Verification items for the finished model (mm, model axes). A direction names the side the tool comes from. Coordinates: 2 decimals unless noted, no trailing zeros. Order: outer loops, then holes, each group sorted by start corner. A loop starts at its lowest first (then second) coordinate and runs counter-clockwise, first axis right, second up. Notation, with made-up numbers: M 61.25,63 L 67.25,63 A21 ccw 67.25,76 Z; hole C 51.5,-37 d5. An arc over 180 degrees is marked long. Write item = value, one per line.
```python
from build123d import *

# Parameters (mm, degrees)
SKETCH1_W                  = 52
SKETCH1_H                  = 28.5
SKETCH1_R                  = 1.6
BOSS_EXTRUDE1_DEPTH        = 1.6
FILLET1_R                  = 2
SKETCH2_W                  = 6
SKETCH2_H                  = 8
BOSS_EXTRUDE2_DEPTH        = 2.6
SKETCH3_W                  = 26.5
SKETCH3_H                  = 18.5
BOSS_EXTRUDE3_DEPTH        = 0.9
SKETCH4_W                  = 19
SKETCH4_H                  = 18.5
BOSS_EXTRUDE4_DEPTH        = 2.4
SKETCH5_W                  = 4.480247742
SKETCH5_H                  = 2.767211841
SKETCH5_H_2                = 2.398250262
BOSS_EXTRUDE5_DEPTH        = 2
CUT_EXTRUDE1_START         = -1.6
CUT_EXTRUDE1_OUTLINE_R     = 1.6
CUT_EXTRUDE1_DEPTH         = 1.6
CUT_EXTRUDE1_2_OUTLINE_W   = 6
CUT_EXTRUDE1_2_OUTLINE_H   = 8
CUT_EXTRUDE1_2_OUTLINE_W_2 = 4.480247742
CUT_EXTRUDE1_2_OUTLINE_H_2 = 2.767211841
CUT_EXTRUDE1_2_OUTLINE_H_3 = 2.398250262
CUT_EXTRUDE1_2_DEPTH       = 2.6


# Read off the part's stored shape, not the designer's step: Cut-Extrude1
with BuildPart() as part:
    # Sketch1 → Boss-Extrude1 (new body)
    with BuildSketch(Plane(origin=(0, 0, 0), x_dir=(1, 0, 0), z_dir=(0, 1, 0))):
        Rectangle(SKETCH1_W, SKETCH1_H)
        with Locations(Location((-23.7, 11.55, 0), (0, 0, 270))):
            Circle(SKETCH1_R, mode=Mode.SUBTRACT)
        with Locations(Location((-23.7, -11.55, 0), (0, 0, 270))):
            Circle(SKETCH1_R, mode=Mode.SUBTRACT)
        with Locations(Location((23.4, 11.55, 0), (0, 0, 270))):
            Circle(SKETCH1_R, mode=Mode.SUBTRACT)
        with Locations(Location((23.4, -11.55, 0), (0, 0, 270))):
            Circle(SKETCH1_R, mode=Mode.SUBTRACT)
    extrude(amount=BOSS_EXTRUDE1_DEPTH)

    # Fillet1
    fillet1_edges = [part.edges().sort_by_distance(p)[0] for p in [
        (-26, 0.8, -14.25),
        (26, 0.8, -14.25),
        (26, 0.8, 14.25),
        (-26, 0.8, 14.25),
    ]]
    fillet(fillet1_edges, radius=FILLET1_R)

    # Sketch2 → Boss-Extrude2 (add)
    with BuildSketch(Plane(origin=(0, 1.6, 0), x_dir=(1, 0, 0), z_dir=(0, 1, 0))):
        with Locations((-23, 0)):
            Rectangle(SKETCH2_W, SKETCH2_H)
    extrude(amount=BOSS_EXTRUDE2_DEPTH)

    # Sketch3 → Boss-Extrude3 (add)
    with BuildSketch(Plane(origin=(0, 1.6, 0), x_dir=(1, 0, 0), z_dir=(0, 1, 0))):
        with Locations((12.75, 0)):
            Rectangle(SKETCH3_W, SKETCH3_H)
    extrude(amount=BOSS_EXTRUDE3_DEPTH)

    # Sketch4 → Boss-Extrude4 (add)
    with BuildSketch(Plane(origin=(0, 2.5, 0), x_dir=(1, 0, 0), z_dir=(0, 1, 0))):
        with Locations((9, 0)):
            Rectangle(SKETCH4_W, SKETCH4_H)
    extrude(amount=BOSS_EXTRUDE4_DEPTH)

    # Sketch5 → Boss-Extrude5 (add)
    with BuildSketch(Plane(origin=(0, 1.6, 0), x_dir=(1, 0, 0), z_dir=(0, 1, 0))):
        with Locations((-23.323642657, 8.222572326)):
            Rectangle(SKETCH5_W, SKETCH5_H)
        with Locations((-23.323642657, -8.459761913)):
            Rectangle(SKETCH5_W, SKETCH5_H_2)
    extrude(amount=BOSS_EXTRUDE5_DEPTH)

    # Cut-Extrude1 outline → Cut-Extrude1 (cut)
    with BuildSketch(Plane(origin=(0, 1.6, 0), x_dir=(1, 0, 0), z_dir=(0, 1, 0)).offset(CUT_EXTRUDE1_START)):
        with BuildLine():
            ThreePointArc((-26, -12.25), (-25.414213562, -13.664213562), (-24, -14.25))
            Line((-24, -14.25), (24, -14.25))
            ThreePointArc((24, -14.25), (25.414213562, -13.664213562), (26, -12.25))
            Line((26, -12.25), (26, 12.25))
            ThreePointArc((26, 12.25), (25.414213562, 13.664213562), (24, 14.25))
            Line((24, 14.25), (-24, 14.25))
            ThreePointArc((-24, 14.25), (-25.414213562, 13.664213562), (-26, 12.25))
            Line((-26, 12.25), (-26, -12.25))
        make_face()
        with Locations((-23.7, -11.55)):
            Circle(CUT_EXTRUDE1_OUTLINE_R, mode=Mode.SUBTRACT)
        with Locations((23.4, -11.55)):
            Circle(CUT_EXTRUDE1_OUTLINE_R, mode=Mode.SUBTRACT)
        with Locations((-23.7, 11.55)):
            Circle(CUT_EXTRUDE1_OUTLINE_R, mode=Mode.SUBTRACT)
        with Locations((23.4, 11.55)):
            Circle(CUT_EXTRUDE1_OUTLINE_R, mode=Mode.SUBTRACT)
    extrude(amount=CUT_EXTRUDE1_DEPTH, mode=Mode.SUBTRACT)

    # Cut-Extrude1 2 outline → Cut-Extrude1 2 (cut)
    with BuildSketch(Plane(origin=(0, 1.6, 0), x_dir=(1, 0, 0), z_dir=(0, 1, 0))):
        with Locations((-23, 0)):
            Rectangle(CUT_EXTRUDE1_2_OUTLINE_W, CUT_EXTRUDE1_2_OUTLINE_H)
        with Locations((-23.323642657, 8.222572326)):
            Rectangle(CUT_EXTRUDE1_2_OUTLINE_W_2, CUT_EXTRUDE1_2_OUTLINE_H_2)
        with Locations((-23.323642657, -8.459761913)):
            Rectangle(CUT_EXTRUDE1_2_OUTLINE_W_2, CUT_EXTRUDE1_2_OUTLINE_H_3)
    extrude(amount=CUT_EXTRUDE1_2_DEPTH, mode=Mode.SUBTRACT)


solid = part.part
```
Item 1: Tool access check on faces 1 (the flat face through (18.5, 4, 0)), 2 (the flat face through (10, 3, 9.25)). Record the directions out of +Z, -Z, +X, -X, +Y, -Y that give a thin tool (end or side, any length) a straight path to the whole face; none if there is none.
Report:
face_1 = +Z, -Z, +X, +Y
face_2 = +Z, +X, -X, +Y, -Y
Item 2: Sectioned sample at B-B, the plane x = 21.75. Enter the section's corners in (y, z), then the cut area to 4 significant figures.
Report:
outline = M 1.6,-9.25 L 2.5,-9.25 L 2.5,9.25 L 1.6,9.25 Z
area = 16.65 mm^2
Item 3: Scan lines: L1, parallel to X at y = 4.4, z = 4.5; L2, parallel to Y at x = 24.25, z = -2. Record each from-to range of solid material in increasing order. Write a range as from..to.
Report:
L1 = -0.5..18.5
L2 = 1.6..2.5
Item 4: Gauge pin test, flat ends, axial feed: pin 1 (0.7 mm diameter, centred on y = 4, z = 2.5, fed in from +X); pin 2 (6 mm diameter, centred on x = 22.5, z = 0, fed in from +Y). Record the tip position at first contact, or that the pin passes through.
Report:
pin_1 = 18.5
pin_2 = 2.5
Item 5: Sectioned sample at C-C, the plane y = 3.95. Enter the section's corners in (x, z).
Report:
outline = M -0.5,-9.25 L 18.5,-9.25 L 18.5,9.25 L -0.5,9.25 Z
Item 6: Sectioned sample at A-A, the plane z = -2.5. Enter the section's corners in (x, y).
Report:
outline = M -0.5,1.6 L 26,1.6 L 26,2.5 L 18.5,2.5 L 18.5,4.9 L -0.5,4.9 Z
